Geometry check sheet. Reference: the model listing, model coordinates, mm. A direction names the side the tool comes from. Coordinates: 2 decimals unless noted, no trailing zeros. Write each loop counter-clockwise with the first axis right and the second up, starting at its lowest first coordinate (ties: lowest second). Pieces come first, ordered by that corner, then holes. Notation, with made-up numbers: (28, 67.25) -> (72, 67.25) arc R9 ccw to (72, 81.25) -> close; hole circle Ø10 at (64, -32). An arc over 180 degrees is marked (long way). Answer in a Markdown table with one row per item. Add a question column.
Q1. Gauge pin test, flat end, axial feed: P1, Ø1.1, axis at x = 12, y = -2, coming from the -Z side. Record the tip position at first contact, or that the pin passes through.
Q2. Thickness scan on line 1 (X direction, y = -2.8, z = 17); line 2 (X direction, y = -2, z = 4); line 3 (Z direction, x = -2.5, y = -2). Record the ranges inside material, lowest first.
Q3. Release check for a two-part mould opening along Z. For faces 1 (the face through (-3.09, -1.88, 27.84)), 2 (the face through (35.31, -1.878, -7.064)), 3 (the face through (20, -3.81, 2)) record: pulls with the +Z half, pulls with the -Z half, needs draft (parallel to the pull), parting line crosses it, or undercut.
Q4. Tool access check on faces 4 (the face through (10.833, -2, 0)), 5 (the face through (40.807, -1.878, 1.44)), 6 (the face through (5.37, -1.88, 1.69)). Record the directions out of +Z, -Z, +X, -X, +Y, -Y that give a thin tool (end or side, any length) a straight path to the whole face; none if there is none.
Q5. Section check C-C, the plane y = -1.8. Count the separate pieces of the cut face and the enclosed holes in it, and give its area (3 significant figures).
Q6. Section check A-A, the plane z = 6.5. Record the boundary of the cut face in (x, y), and give its area (3 significant figures).
Q7. Section check B-B, the plane x = 32. Record the boundary of the cut face in (y, z).
```python
from build123d import *

# Parameters (mm, degrees)
F1_DEPTH = 3.81
F2_R     = 0.254
F3_D     = 1.778


# Not quite as in the source:
# - a feature names something its author has since deleted; it is built from what else it names


with BuildPart() as f1:
    # F0 (on Front) → F1 (new body)
    with BuildSketch(Plane.XZ):
        with BuildLine():
            ThreePointArc((41.4086468518, -4.477661373), (40.8064485211, 1.5249027452), (41.4086468518, 7.5274668634))
            ThreePointArc((41.4086468518, 7.5274668634), (38.62243375, 10.6323405578), (35.8362206482, 7.5274668634))
            ThreePointArc((35.8362206482, 7.5274668634), (26.9629642945, 0.6052852493), (18.0897079408, 7.5274668634))
            ThreePointArc((18.0897079408, 7.5274668634), (16.3997087002, 8.5658356165), (14.7097094595, 7.5274668634))
            ThreePointArc((14.7097094595, 7.5274668634), (5.20431123, 1.6871633473), (-4.3010869995, 7.5274668634))
            ThreePointArc((-4.3010869995, 7.5274668634), (-5.8660457098, 16.6021063924), (-4.3010869995, 25.6767459214))
            ThreePointArc((-4.3010869995, 25.6767459214), (-3.0718420066, 27.8672574596), (-1.3499599881, 29.6960566193))
            ThreePointArc((-1.3499599881, 29.6960566193), (-0.1811880249, 31.805372823), (-0.6376186502, 34.1732650995))
            ThreePointArc((-0.6376186502, 34.1732650995), (-1.421034245, 31.7066061173), (-2.9725597706, 29.6351537108))
            ThreePointArc((-2.9725597706, 29.6351537108), (-4.1943946694, 27.9789305778), (-5.8506173082, 26.7570950091))
            ThreePointArc((-5.8506173082, 26.7570950091), (-7.277149178, 25.8612568479), (-8.1605734304, 24.4270041585))
            ThreePointArc((-8.1605734304, 24.4270041585), (-7.1141917577, 19.7155957013), (-6.9871647283, 14.8910596211))
            Line((-6.9871647283, 14.8910596211), (-6.5609117303, 7.4617798516))
            Line((-6.5609117303, 7.4617798516), (-5.4928543977, 4.8075970262))
            Line((-5.4928543977, 4.8075970262), (-4.555047024, 4.7773430124))
            Line((-4.555047024, 4.7773430124), (-4.4945431873, 2.3267425131))
            Line((-4.4945431873, 2.3267425131), (-5.734869279, 2.2662337869))
            ThreePointArc((-5.734869279, 2.2662337869), (-1.646496666, 0.760301383), (2.5915002188, -0.2506414603))
            Line((2.5915002188, -0.2506414603), (10.8333304524, -0.2506414603))
            Line((10.8333304524, -0.2506414603), (10.8333304524, 0.9162292117))
            Line((10.8333304524, 0.9162292117), (12.9701783881, 0.9162292117))
            Line((12.9701783881, 0.9162292117), (12.9701783881, -0.2506414603))
            Line((12.9701783881, -0.2506414603), (15.6823657453, -0.8442893741))
            ThreePointArc((15.6823657453, -0.8442893741), (18.751499307, -2.5127162084), (21.4028581977, -4.7872546129))
            ThreePointArc((21.4028581977, -4.7872546129), (22.004430538, -6.2762052491), (21.9660382718, -7.8816302121))
            Line((21.9660382718, -7.8816302121), (28.9244800806, -7.9146586359))
            ThreePointArc((28.9244800806, -7.9146586359), (35.3988018628, -7.0397169385), (41.4086468518, -4.477661373))
        make_face()
    extrude(amount=F1_DEPTH)

    # F2
    f2_edges = [f1.edges().sort_by_distance(p)[0] for p in [
        (-0.637619, -1.905, 34.173265),
        (21.966038, -1.905, -7.88163),
        (-5.734869, -1.905, 2.266234),
    ]]
    fillet(f2_edges, radius=F2_R)

    # F3 (through all)
    with Locations(Plane(origin=(0, 0, 0), x_dir=(1, 0, 0), z_dir=(0, 1, 0))):
        with Locations((28.9652328938, 3.4148474224), (-6.2686339952, -24.3659485132)):
            Hole(F3_D / 2)


solid = f1.part
```
Calculated:
| question | item | result |
|---|---|---|
| 1 | P1 | stops at z = 0.92 |
| 2 | line 1 | x = -6.93 to -5.86 |
| 2 | line 2 | x = -4.54 to -1.42, 11.83 to 19.85, 34.08 to 40.91 |
| 2 | line 3 | z = 1.03 to 4.98, 28.58 to 30.13 |
| 3 | face 1 | undercut |
| 3 | face 2 | pulls with the -Z half |
| 3 | face 3 | needs draft |
| 4 | face 4 | -Z, +Y, -Y |
| 4 | face 5 | +X, +Y, -Y |
| 4 | face 6 | +Y, -Y |
| 5 | separate pieces | 1 |
| 5 | enclosed holes | 2 |
| 5 | area | 384 mm² |
| 6 | outline | (-6.17, -3.81) -> (-3.71, -3.81) -> (-3.71, 0) -> (-6.17, 0) -> close; (14.12, -3.81) -> (18.41, -3.81) -> (18.41, 0) -> (14.12, 0) -> close; (35.51, -3.81) -> (41.22, -3.81) -> (41.22, 0) -> (35.51, 0) -> close |
| 6 | area | 47.5 mm² |
| 7 | outline | (-3.81, -7.72) -> (0, -7.72) -> (0, 2.12) -> (-3.81, 2.12) -> close |
